Geometry check sheet. Reference: the model listing, model coordinates, mm. Face numbers are marked on the shaded views. Round coordinates to 2 decimals unless told otherwise and drop trailing zeros. Write each loop counter-clockwise with the first axis right and the second up, starting at its lowest first coordinate (ties: lowest second). Pieces come first, ordered by that corner, then holes. Notation, with made-up numbers: (27.5, 28) -> (51.5, 28) arc R26 cw to (51.5, 55) -> close; hole circle Ø2 at (42.25, -22.75). An arc over 180 degrees is marked (long way). One line per question, with ' | ' between items.
```python
from build123d import *

# Parameters (mm, degrees)
F0_R         = 19.05
F1_DEPTH     = 2.54
F2_R         = 3.175
F3_DEPTH     = 44.45
F4_R         = 9.525
F5_DEPTH     = 1.27
F6_R         = 3.175
F7_DEPTH     = 5.08
F8_R         = 15.875
F9_DEPTH     = 3.81
F10_S5_R     = 3.175
F10_T6_DEPTH = 24


# Not quite as in the source:
# - a fillet or chamfer that OpenCascade refuses, or shapes differently, is made with other operations: its cross-section is extruded or revolved along the edge and cut away or added


with BuildPart() as f1:
    # F0 (on Top) → F1 (new body)
    with BuildSketch(Plane.XY):
        Circle(F0_R)
    extrude(amount=F1_DEPTH)

    # F2 (on face) → F3 (join)
    with BuildSketch(Plane(origin=(0, 0, 0), x_dir=(1, 0, 0), z_dir=(0, 0, -1))):
        Circle(F2_R)
    extrude(amount=F3_DEPTH)

    # F4 (on face) → F5 (join)
    with BuildSketch(Plane(origin=(0, 0, -44.45), x_dir=(1, 0, 0), z_dir=(0, 0, -1))):
        Circle(F4_R)
    extrude(amount=F5_DEPTH)

    # F6 (on face) → F7 (join)
    with BuildSketch(Plane(origin=(0, 0, -45.72), x_dir=(1, 0, 0), z_dir=(0, 0, -1))):
        Circle(F6_R)
    extrude(amount=F7_DEPTH)

    # F8 (on face) → F9 (join)
    with BuildSketch(Plane(origin=(0, 0, -50.8), x_dir=(1, 0, 0), z_dir=(0, 0, -1))):
        Circle(F8_R)
    extrude(amount=F9_DEPTH)

    # F10: chamfer of 2.54 x 14.4050558218 on 1 edges, made by hand


with BuildPart() as f10_tool2:
    # F10_s3 → F10_t4 (revolve)
    with BuildSketch(Plane.XZ):
        Polygon((15.875, -53.34), (1.4699441782, -50.8), (15.875, -50.8), align=None)
    revolve(axis=Axis((0, 0, -50.8), (0, 0, -1)))

    # F10_s5 → F10_t6 (cut, symmetric)
    with BuildSketch(Plane.XY.offset(-52.1)):
        Circle(F10_S5_R)
    extrude(amount=F10_T6_DEPTH, both=True, mode=Mode.SUBTRACT)


with BuildPart() as f1_1:
    add(f1.part)

    # F10_t1: cut F10_tool2
    add(f10_tool2.part, mode=Mode.SUBTRACT)


solid = f1_1.part
```
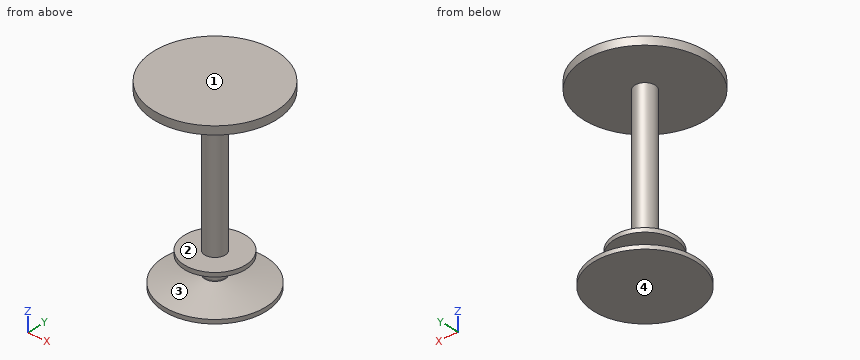
(1) Sectioned sample at A-A on y = 0. Record the cut outline in (x, z) (3 decimals).
Resolved:
outline: (-19.05, 0) -> (-3.175, 0) -> (-3.175, -44.45) -> (-9.525, -44.45) -> (-9.525, -45.72) -> (-3.175, -45.72) -> (-3.175, -51.101) -> (-15.875, -53.34) -> (-15.875, -54.61) -> (15.875, -54.61) -> (15.875, -53.34) -> (3.175, -51.101) -> (3.175, -45.72) -> (9.525, -45.72) -> (9.525, -44.45) -> (3.175, -44.45) -> (3.175, 0) -> (19.05, 0) -> (19.05, 2.54) -> (-19.05, 2.54) -> close
(2) Go/stop test with a flat-tipped pin: pin 1 (10 mm diameter, centred on y = 5, z = -46, fed in from -X) (3 decimals). Record where the tip stops, or that it passes through.
Resolved:
pin 1: stops at x = -9.525
(3) Sectioned sample at D-D on z = -15.5. Record the cut outline in (x, y) (3 decimals), then the cut area to 3 significant figures.
Resolved:
outline: circle Ø6.35 at (0, 0) | area: 31.7 mm2
(4) Sectioned sample at C-C on y = 6. Count the separate pieces of the cut face and the enclosed holes in it, then the cut area to 3 significant figures.
Resolved:
separate pieces: 3 | enclosed holes: 0 | area: 179 mm2
(5) Material ranges on line 1 (Z direction, x = 1, y = -4.5); line 2 (Z direction, x = -8, y = -14.5); line 3 (Z direction, x = -15, y = -3.5), recorded low to high.
Resolved:
line 1: z = -54.61 to -51.35, -45.72 to -44.45, 0 to 2.54 | line 2: z = 0 to 2.54 | line 3: z = -54.61 to -53.26, 0 to 2.54
(6) Draft check along Z on the marked faces 1, 2, 3 and 4. Enter one of: +Z half, -Z half, draft (parallel to the pull), parting line (faces both ways), or undercut.
Resolved:
face 1: +Z half | face 2: undercut | face 3: undercut | face 4: -Z half
